Can you work these out from the model? Positions are in its coordinate system, mm. A direction names the side the tool comes from. Round coordinates to 2 decimals unless told otherwise and drop trailing zeros. Order: outer loops, then holes, each group sorted by start corner. A loop starts at its lowest first (then second) coordinate and runs counter-clockwise, first axis right, second up. Notation, with made-up numbers: M -3,69.5 L 34,69.5 A15 ccw 34,74.5 Z; hole C -20.5,-32 d7. An arc over 180 degrees is marked long. Answer as a JSON object with one key per item and string values. Group by question number.
from build123d import *

# Parameters (mm, degrees)
Y_KSEKLIK_EKSTR_ZYON1_DEPTH = 100
IZIM2_W                     = 42
IZIM2_H                     = 60
KES_EKSTR_ZYON1_DEPTH       = 15
IZIM3_R                     = 4
IZIM3_R_2                   = 3
KES_EKSTR_ZYON2_DEPTH       = 175.685863047
IZIM4_R                     = 7.5
KES_EKSTR_ZYON5_DEPTH       = 175.685863047
IZIM5_R                     = 9
KES_EKSTR_ZYON6_DEPTH       = 226.427594277


with BuildPart() as part:
    # Çizim1 → Yükseklik-Ekstrüzyon1 (new body)
    with BuildSketch(Plane(origin=(0, 0, 0), x_dir=(0, 0, -1), z_dir=(1, 0, 0))):
        Polygon((-127.632874873, 26.747480954), (-127.632874873, 6.747480954), (77.367125127, 6.747480954), (77.367125127, 21.747480954), (52.367125127, 21.747480954), (52.367125127, 91.747480954), (32.367125127, 91.747480954), (32.367125127, 41.747480954), (-27.632874873, 41.747480954), (-27.632874873, 26.747480954), align=None)
    extrude(amount=Y_KSEKLIK_EKSTR_ZYON1_DEPTH)

    # Çizim2 → Kes-Ekstrüzyon1 (cut)
    with BuildSketch(Plane(origin=(0, 41.747480954, 0), x_dir=(1, 0, 0), z_dir=(0, 1, 0))):
        with Locations((50, 2.367125127)):
            Rectangle(IZIM2_W, IZIM2_H)
    extrude(amount=-KES_EKSTR_ZYON1_DEPTH, mode=Mode.SUBTRACT)

    # Çizim3 → Kes-Ekstrüzyon2 (cut, through all)
    with BuildSketch(Plane(origin=(0, 26.747480954, 0), x_dir=(1, 0, 0), z_dir=(0, 1, 0))):
        with Locations(Location((15, 64.867125127, 0), (0, 0, 270))):
            Circle(IZIM3_R)
        with Locations(Location((85, 64.867125127, 0), (0, 0, 270))):
            Circle(IZIM3_R)
        with Locations(Location((33, -105.132874873, 0), (0, 0, 270))):
            Circle(IZIM3_R_2)
        with Locations(Location((67, -105.132874873, 0), (0, 0, 270))):
            Circle(IZIM3_R_2)
    extrude(amount=-KES_EKSTR_ZYON2_DEPTH, mode=Mode.SUBTRACT)

    # Çizim4 → Kes-Ekstrüzyon5 (cut, through all)
    with BuildSketch(Plane(origin=(0, 26.747480954, 0), x_dir=(1, 0, 0), z_dir=(0, 1, 0))):
        with Locations(Location((15, -45.632874873, 0), (0, 0, 270))):
            Circle(IZIM4_R)
        with Locations(Location((85, -45.632874873, 0), (0, 0, 270))):
            Circle(IZIM4_R)
    extrude(amount=-KES_EKSTR_ZYON5_DEPTH, mode=Mode.SUBTRACT)

    # Çizim5 → Kes-Ekstrüzyon6 (cut, through all)
    with BuildSketch(Plane(origin=(0, 0, -52.367125127), x_dir=(-1, 0, 0), z_dir=(0, 0, -1))):
        with Locations((-50, 51.747480954)):
            Circle(IZIM5_R)
    extrude(amount=-KES_EKSTR_ZYON6_DEPTH, mode=Mode.SUBTRACT)


solid = part.part
Item 1: Suppose I cut it at B-B, the plane x = 50. Write out the boundary of the cut face in (y, z).
Item 2: If we mould it in two halves opening along X, with no side actions, what happens to faces 5 (the face through (14, 34, 27.633)), 6 (the face through (0, 31, 4)), 7 (the face through (65.175, 16.887, 102.752))? For each: +X half, -X half, draft (parallel to the pull), parting line (faces both ways), or undercut.
Item 3: Suppose I cut it at D-D, the plane y = 46.5. Write out the boundary of the cut face in (x, z), and give its area (3 significant figures).
Item 4: I'm going to push flat-ended pins straight in: pin 1 Ø10 at (x, y) = (55, 42.5) entering from -Z; pin 2 Ø14.5 at (x, z) = (20.5, -8.5) entering from +Y; pin 3 Ø1 at (x, y) = (23.5, 64) entering from +Z; pin 4 Ø16.5 at (y, z) = (35, -17.5) entering from -X. Where does each tip first touch, or does it pass through?
Item 5: On a 3-axis mill with a long thin cutter (end or side, diameter ignored), from which of +Z, -Z, +X, -X, +Y, -Y can I reach the whole of each face in a straight line? I mean faces 1 (the face through (49, 21.747, -65)), 2 (the face through (100, 31, 4)), 3 (the face through (71, 34, -2)), 4 (the face through (14, 41.747, -3)). Say none if no direction works.
Item 6: Suppose I cut it at A-A, the plane x = 85. Write out the boundary of the cut face in (y, z).
Item 7: Suppose I cut it at C-C, the plane y = 18. Write out the boundary of the cut face in (x, z), and give its area (3 significant figures).
Item 8: I need wall thicknesses on line 1 (Z direction, x = 24, y = 42); line 2 (Y direction, x = 51.5, z = 91); line 3 (Y direction, x = 8.5, z = -53.5). Which ranges of each line are inside material? Lowest first, please.
Computed:
{
 "1": {"outline": "M 6.75,-77.37 L 21.75,-77.37 L 21.75,-52.37 L 42.75,-52.37 L 42.75,-32.37 L 26.75,-32.37 L 26.75,127.63 L 6.75,127.63 Z; M 60.75,-52.37 L 91.75,-52.37 L 91.75,-32.37 L 60.75,-32.37 Z"},
 "2": {"face 5": "draft", "face 6": "-X half", "face 7": "undercut"},
 "3": {"outline": "M 0,-52.37 L 42.69,-52.37 L 42.69,-32.37 L 0,-32.37 Z; M 57.31,-52.37 L 100,-52.37 L 100,-32.37 L 57.31,-32.37 Z", "area": "1,710 mm^2"},
 "4": {"pin 1": "stops at z = -52.37", "pin 2": "stops at y = 41.75", "pin 3": "stops at z = -32.37", "pin 4": "stops at x = 0"},
 "5": {"face 1": "-Z, +X, -X, +Y", "face 2": "+Z, -Z, +X, +Y, -Y", "face 3": "+Z, +Y", "face 4": "+Z, +X, -X, +Y"},
 "6": {"outline": "M 6.75,-77.37 L 21.75,-77.37 L 21.75,-68.87 L 6.75,-68.87 Z; M 6.75,-60.87 L 21.75,-60.87 L 21.75,-52.37 L 91.75,-52.37 L 91.75,-32.37 L 41.75,-32.37 L 41.75,27.63 L 26.75,27.63 L 26.75,38.13 L 6.75,38.13 Z; M 6.75,53.13 L 26.75,53.13 L 26.75,127.63 L 6.75,127.63 Z"},
 "7": {"outline": "M 0,-77.37 L 100,-77.37 L 100,127.63 L 0,127.63 Z; hole C 15,45.63 d15; hole C 15,-64.87 d8; hole C 33,105.13 d6; hole C 67,105.13 d6; hole C 85,45.63 d15; hole C 85,-64.87 d8", "area": "20,000 mm^2"},
 "8": {"line 1": "z = -52.37 to -32.37", "line 2": "y = 6.75 to 26.75", "line 3": "y = 6.75 to 21.75"}
}
